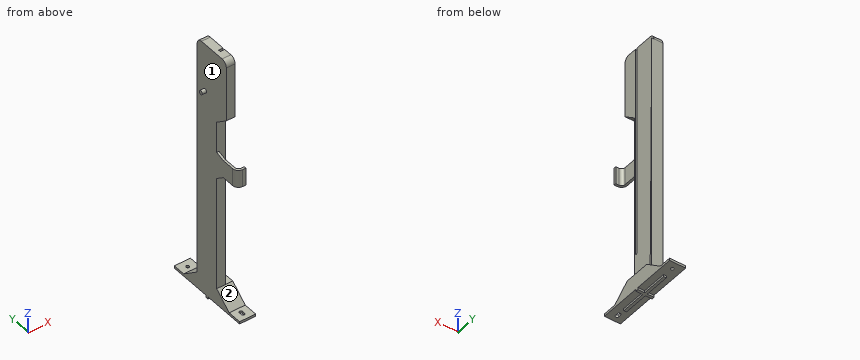
```python
from build123d import *

# Parameters (mm, degrees)
BOSS_EXTRUDE1_DEPTH  = 12.6
BOSS_EXTRUDE2_DEPTH  = 23.1
BOSS_EXTRUDE3_DEPTH  = 3.175
SKETCH1_5_W          = 25.4
SKETCH1_5_H          = 3.175
BOSS_EXTRUDE4_DEPTH  = 12.7
FILLET1_R            = 5
FILLET2_R            = 8.175
CUT_EXTRUDE1_DEPTH   = 6.35
CUT_EXTRUDE2_REACH   = 386.06
SKETCH3_R            = 2.275
SKETCH4_W            = 23.1
SKETCH4_H            = 3.8
SKETCH4_W_2          = 3.8
SKETCH4_H_2          = 76.45
EXTRUDE_THIN1_DEPTH  = 3.15
SKETCH5_R            = 2.875
BOSS_EXTRUDE5_DEPTH  = 6.2
BOSS_EXTRUDE5_TAPER  = 2
FILLET1_OF_MIRROR1_R = 5
FILLET2_OF_MIRROR1_R = 8.175
SKETCH6_R            = 2.875
BOSS_EXTRUDE6_DEPTH  = 6.2
BOSS_EXTRUDE7_DEPTH  = 3.28


with BuildPart() as part:
    # Sketch1 → Boss-Extrude1 (new body)
    with BuildSketch(Plane(origin=(0, 0, 0), x_dir=(0, 0, -1), z_dir=(1, 0, 0))):
        Polygon((175.575, -37.35), (175.575, 0), (-175.575, 0), (-175.575, -55.88), (-88.271480231, -55.88), (-73.904922854, -37.35), (-28.686383268, -37.35), (10.475, -37.35), align=None)
    boss_extrude1 = extrude(amount=-BOSS_EXTRUDE1_DEPTH)

    # Sketch1<3> → Boss-Extrude2 (add)
    with BuildSketch(Plane(origin=(0, 0, 0), x_dir=(0, 0, -1), z_dir=(1, 0, 0))):
        Polygon((175.575, 0), (195.675, 25.925), (195.675, 43.925), (199.075, 43.925), (199.075, -81.275), (195.675, -81.275), (195.675, -61.275), (175.575, -37.35), align=None)
    boss_extrude2 = extrude(amount=-BOSS_EXTRUDE2_DEPTH)

    # Sketch1<4> → Boss-Extrude3 (add)
    with BuildSketch(Plane(origin=(0, 0, 0), x_dir=(0, 0, -1), z_dir=(1, 0, 0))):
        Polygon((0.628519769, -50.05), (10.475, -37.35), (-28.686383268, -37.35), (-24.771480231, -50.05), (-24.771480231, -73.025), (0.628519769, -73.025), align=None)
    boss_extrude3 = extrude(amount=-BOSS_EXTRUDE3_DEPTH)

    # Sketch1<5> → Boss-Extrude4 (add)
    with BuildSketch(Plane(origin=(0, 0, 0), x_dir=(0, 0, -1), z_dir=(1, 0, 0))):
        with Locations((-12.071480231, -74.6125)):
            Rectangle(SKETCH1_5_W, SKETCH1_5_H)
    boss_extrude4 = extrude(amount=-BOSS_EXTRUDE4_DEPTH)

    # Fillet1
    fillet1_edges = [part.edges().sort_by_distance(p)[0] for p in [
        (-3.175, -73.025, 12.071480231),
    ]]
    fillet(fillet1_edges, radius=FILLET1_R)

    # Fillet2
    fillet2_edges = [part.edges().sort_by_distance(p)[0] for p in [
        (-6.3, -55.88, 175.575),
        (-6.3, 0, 175.575),
        (0, -76.2, 12.071480231),
    ]]
    fillet(fillet2_edges, radius=FILLET2_R)

    # Sketch2 → Cut-Extrude1 (cut)
    with BuildSketch(Plane.ZY.offset(12.6)):
        with BuildLine():
            Line((-131.125, -32.5875), (222.402046917, -32.5875))
            ThreePointArc((222.402046917, -32.5875), (223.989546917, -34.175), (222.402046917, -35.7625))
            Line((222.402046917, -35.7625), (-131.125, -35.7625))
            ThreePointArc((-131.125, -35.7625), (-132.7125, -34.175), (-131.125, -32.5875))
        make_face()
    cut_extrude1 = extrude(amount=-CUT_EXTRUDE1_DEPTH, mode=Mode.SUBTRACT)

    # Sketch3 → Cut-Extrude2 (cut, up to next)
    with BuildSketch(Plane(origin=(0, 0, -199.075), x_dir=(-1, 0, 0), z_dir=(0, 0, -1)), mode=Mode.PRIVATE) as cut_extrude2_sk1:
        with Locations((11.55, 33.65)):
            Circle(SKETCH3_R)
    cut_extrude2_tool1 = extrude(cut_extrude2_sk1.sketch, amount=-CUT_EXTRUDE2_REACH, mode=Mode.PRIVATE) & part.part
    # Sketch3 → Cut-Extrude2 (cut, up to next)
    with BuildSketch(Plane(origin=(0, 0, -199.075), x_dir=(-1, 0, 0), z_dir=(0, 0, -1)), mode=Mode.PRIVATE) as cut_extrude2_sk2:
        with BuildLine():
            Line((9.3, -72.325), (9.3, -68.275))
            ThreePointArc((9.3, -68.275), (11.55, -66.025), (13.8, -68.275))
            Line((13.8, -68.275), (13.8, -72.325))
            ThreePointArc((13.8, -72.325), (11.55, -74.575), (9.3, -72.325))
        make_face()
    cut_extrude2_tool2 = extrude(cut_extrude2_sk2.sketch, amount=-CUT_EXTRUDE2_REACH, mode=Mode.PRIVATE) & part.part
    cut_extrude2_1 = cut_extrude2_tool1.solids().sort_by_distance((-11.55, 33.65, -199.075))[0]
    add(cut_extrude2_1, mode=Mode.SUBTRACT)
    cut_extrude2_2 = cut_extrude2_tool2.solids().sort_by_distance((-11.55, -70.3, -199.075))[0]
    add(cut_extrude2_2, mode=Mode.SUBTRACT)
    cut_extrude2 = cut_extrude2_1 + cut_extrude2_2  # Cut-Extrude2 as one shape, for the pattern or mirror that repeats it

    # Sketch4 → Extrude-Thin1 (add)
    with BuildSketch(Plane(origin=(0, 0, -199.075), x_dir=(-1, 0, 0), z_dir=(0, 0, -1))):
        with Locations((11.55, -18.675)):
            Rectangle(SKETCH4_W, SKETCH4_H)
        with Locations((11.55, -18.675)):
            Rectangle(SKETCH4_W_2, SKETCH4_H_2)
    extrude_thin1 = extrude(amount=EXTRUDE_THIN1_DEPTH)

    # Sketch5 → Boss-Extrude5 (add)
    with BuildSketch(Plane(origin=(0, 0, 0), x_dir=(0, 0, -1), z_dir=(1, 0, 0))):
        with Locations((-106.425, -48.98)):
            Circle(SKETCH5_R)
    extrude(amount=BOSS_EXTRUDE5_DEPTH, taper=BOSS_EXTRUDE5_TAPER)


with BuildPart() as mirror1_1:
    # Mirror1: Boss-Extrude1, Boss-Extrude2, Boss-Extrude3, Boss-Extrude4 across plane
    add(boss_extrude1.mirror(Plane(origin=(0, 0, 0), x_dir=(0, 0, 1), z_dir=(1, 0, 0))))
    add(boss_extrude2.mirror(Plane(origin=(0, 0, 0), x_dir=(0, 0, 1), z_dir=(1, 0, 0))))
    add(boss_extrude3.mirror(Plane(origin=(0, 0, 0), x_dir=(0, 0, 1), z_dir=(1, 0, 0))))
    add(boss_extrude4.mirror(Plane(origin=(0, 0, 0), x_dir=(0, 0, 1), z_dir=(1, 0, 0))))

    # Mirror1 2: Cut-Extrude1, Cut-Extrude2 across plane
    add(cut_extrude1.mirror(Plane(origin=(0, 0, 0), x_dir=(0, 0, 1), z_dir=(1, 0, 0))), mode=Mode.SUBTRACT)
    add(cut_extrude2.mirror(Plane(origin=(0, 0, 0), x_dir=(0, 0, 1), z_dir=(1, 0, 0))), mode=Mode.SUBTRACT)

    # Fillet1 of Mirror1
    fillet1_of_mirror1_edges = [mirror1_1.edges().sort_by_distance(p)[0] for p in [
        (3.175, -73.025, 12.071480231),
    ]]
    fillet(fillet1_of_mirror1_edges, radius=FILLET1_OF_MIRROR1_R)

    # Fillet2 of Mirror1
    fillet2_of_mirror1_edges = [mirror1_1.edges().sort_by_distance(p)[0] for p in [
        (6.3, -55.88, 175.575),
        (6.3, 0, 175.575),
        (0, -76.2, 12.071480231),
    ]]
    fillet(fillet2_of_mirror1_edges, radius=FILLET2_OF_MIRROR1_R)


with BuildPart() as mirror1_3_1:
    # Mirror1 3: Extrude-Thin1 across plane
    add(extrude_thin1.mirror(Plane(origin=(0, 0, 0), x_dir=(0, 0, 1), z_dir=(1, 0, 0))))


with BuildPart() as part_1:
    add(part.part)

    # Mirror1 united with what the copies touc: union Mirror1_1, Mirror1 3_1
    add(mirror1_1.part)
    add(mirror1_3_1.part)

    # SurfaceCut1
    split(bisect_by=Plane(origin=(0, 0, 0), x_dir=(0, 0, -1), z_dir=(1, 0, 0)), keep=Keep.TOP)

    # Sketch6 → Boss-Extrude6 (add)
    with BuildSketch(Plane.ZY):
        with Locations(Location((106.425, -15.125, 0), (0, 0, 180))):
            Circle(SKETCH6_R)
    extrude(amount=BOSS_EXTRUDE6_DEPTH)

    # Sketch7 → Boss-Extrude7 (add)
    with BuildSketch(Plane(origin=(12.6, 0, 0), x_dir=(0, 0, -1), z_dir=(1, 0, 0))):
        Polygon((175.575, 0), (175.575, -3), (-167.4, 0), align=None)
    extrude(amount=BOSS_EXTRUDE7_DEPTH)


solid = part_1.part
```
The model under review builds one solid part; all positions refer to its coordinate system, in mm. Face numbers are marked on the shaded views. Round coordinates to 2 decimals unless told otherwise and drop trailing zeros. Loops run counter-clockwise (first coordinate to the right, second up) from the corner with the lowest first, then second, coordinate; pieces in that order, holes last.
1) Consider section D-D on z = 38.5. State the section outline as (x, y) points, then the cut area to 3 significant figures.
Values follow:
outline: (0, -37.35) - (12.6, -37.35) - (12.6, -35.76) - (6.25, -35.76) - (6.25, -32.59) - (12.6, -32.59) - (12.6, -1.13) - (15.88, -1.13) - (15.88, 0) - (0, 0) - close
area: 454 mm2
2) Consider section B-B on z = -14. State the section outline as (x, y) points.
Values follow:
outline: (0, -37.35) - (12.6, -37.35) - (12.6, -35.76) - (6.25, -35.76) - (6.25, -32.59) - (12.6, -32.59) - (12.6, -1.59) - (15.88, -1.59) - (15.88, 0) - (0, 0) - close
3) Consider section A-A on y = -41.5. State the section outline as (x, z) points (3 decimals).
Values follow:
outline: (0, -199.075) - (9.65, -199.075) - (9.65, -202.225) - (13.45, -202.225) - (13.45, -199.075) - (23.1, -199.075) - (23.1, -179.062) - (0, -179.062) - close; (0, -7.257) - (3.175, -7.257) - (3.175, 27.407) - (0, 27.407) - close; (0, 77.122) - (12.6, 77.122) - (12.6, 175.575) - (0, 175.575) - close
4) Wall thickness on line 1 along Y through (x, z) = (11.55, -198.05) (3 decimals); line 2 along Z through (x, y) = (2.25, -66) (3 decimals); line 3 along X through (y, z) = (33, -197): over which ranges is each line inside the solid? List them lowest first.
Values follow:
line 1: y = -81.275 to -74.575, -66.025 to 31.375, 35.925 to 43.925
line 2: z = -199.075 to -195.675, -0.629 to 24.771
line 3: x = 0 to 9.37, 13.73 to 23.1
5) The part is to be moulded in two halves that separate along Z. For the marked faces 1 and 2, say which applies: pulls with the +Z half, pulls with the -Z half, needs draft (parallel to the pull), parting line crosses it, or undercut.
Values follow:
face 1: needs draft
face 2: undercut
6) Clearance check with flat-ended pins moving along their axes: P1, Ø3, axis at x = 17.5, y = -30, coming from the -Z side (3 decimals); P2, Ø10, axis at x = 3, y = -58.5, coming from the +Z side; P3, Ø12, axis at y = 2, z = 130, coming from the +X side; P4, Ø3.5, axis at x = 4.5, z = -200, coming from the +Y side (3 decimals). State where each tip first meets the part, or that it passes through.
Values follow:
P1: stops at z = -199.075
P2: stops at z = 173.17
P3: stops at x = 15.88
P4: stops at y = 43.925
7) Consider section C-C on y = 15. State the section outline as (x, z) points (3 decimals).
Values follow:
outline: (0, -199.075) - (9.65, -199.075) - (9.65, -202.225) - (13.45, -202.225) - (13.45, -199.075) - (23.1, -199.075) - (23.1, -187.205) - (0, -187.205) - close
